Autodesk Inventor part; units mm, degrees
ref_plane "YZ Plane" through (0, 0, 0) normal (1, 0, 0) x (0, 1, 0)
ref_plane "XZ Plane" through (0, 0, 0) normal (0, 1, 0) x (-1, 0, 0)
ref_plane "XY Plane" through (0, 0, 0) normal (0, 0, 1) x (1, 0, 0)
sketch "Szkic1" plane through (0, 0, 0) normal (0, 0, 1) x (1, 0, 0)
  line L0 (-15.1556, -3.6171) -> (-15.1556, -6.6171)
  line L1 (-15.1556, -6.6171) -> (16.3444, -6.6171)
  line L2 (16.3444, -6.6171) -> (16.3444, 13.3829)
  line L3 (16.3444, 13.3829) -> (13.3444, 13.3829)
  line L4 (13.3444, 13.3829) -> (13.3444, -3.6171)
  line L5 (13.3444, -3.6171) -> (-15.1556, -3.6171)
  point P0 (0, 0)
  dimension "d0" = 3
  dimension "d1" = 31.5
  dimension "d2" = 20
  dimension "d3" = 3
extrude "Wyciągnięcie proste1" add sketch "Szkic1" along normal blind 40
fillet "Zaokrąglenie1" radius 3 1 edges at (13.3444, -3.6171, 20)
fillet "Zaokrąglenie3" radius 2 2 edges at (14.8444, 13.3829, 40) (14.8444, 13.3829, 0)
sketch "Szkic4" plane through (-15.1556, -6.6171, 0) normal (0, -1, 0) x (1, 0, 0)
  line L0 (0, 0) -> (31.5, 0)
  line L1 (31.5, 0) -> (31.5, 40)
  line L2 (0, 40) -> (31.5, 40)
  line L3 (0, 0) -> (0, 40)
  line L4 (31.5, 36.2) -> (-0.3213, 36.2)
  line L5 (31.5, 2) -> (31.5, 38)
  line L6 (31.5, 3.8) -> (0, 3.8)
  line L7 (0, 0) -> (0, 40)
  line L8 (27, 36.2) -> (27, 3.8)
  point P0 (15.1556, 0)
  point P1 (23.5, 30)
  point P2 (3.5, 30)
  point P3 (23.5, 10)
  point P4 (3.5, 10)
  dimension "d47" = 32.4
  dimension "d48" = 3.8
  dimension "d50" = 3.5
  dimension "d51" = 3.5
  dimension "d53" = 6.2
  dimension "d54" = 6.2
  dimension "d55" = 6.2
  dimension "d56" = 6.2
  dimension "d68" = 4.5
  dimension "d69" = 3.5
  dimension "d70" = 3.5
  dimension "d78" = 27
sketch "Szkic5" plane through (16.3444, -6.6171, 40) normal (1, 0, 0) x (0, 0, -1)
  arc A0 (40, 18) -> (38, 20) centre (38, 18) ccw
  line L0 (38, 20) -> (2, 20)
  arc A1 (2, 20) -> (0, 18) centre (2, 18) ccw
  line L1 (0, 0) -> (0, 18)
  line L2 (40, 0) -> (0, 0)
  line L3 (40, 0) -> (40, 18)
  point P0 (40, 6.6171)
  point P1 (10, 10)
  point P2 (30, 10)
  dimension "d57" = 10
  dimension "d58" = 10
  dimension "d59" = 10
  dimension "d60" = 10
hole "Otwór3" at (16.3444, 3.3829, 30) at (16.3444, 3.3829, 10) direction (-1, 0, 0) diameter 5 end through all
hole "Otwór4" at (8.3444, -6.6171, 30) at (-11.6556, -6.6171, 30) at (8.3444, -6.6171, 10) at (-11.6556, -6.6171, 10) direction (0, 1, 0) diameter 3 end through all
sketch "Szkic6" plane through (-15.1556, -3.6171, 40) normal (0, 1, 0) x (1, 0, 0)
  circle A0 centre (23.5, 10) radius 1.5
  circle A1 centre (23.5, 30) radius 1.5
  circle A2 centre (23.5, 10) radius 1.5
  circle A3 centre (23.5, 10) radius 3.1
  circle A4 centre (23.5, 30) radius 3.1
  point P0 (15.1556, 40)
  dimension "d79" = 6.2
  dimension "d80" = 6.2
extrude "Wyciągnięcie proste3" cut sketch "Szkic6" along normal blind 10
chamfer "Faza3" distance 4 angle 45 2 edges at (-15.1556, -5.1171, 40) (-15.1556, -5.1171, 0)
fillet "Zaokrąglenie4" radius 2 4 edges at (-15.1556, -5.1171, 36) (-11.1556, -5.1171, 40) (-15.1556, -5.1171, 4) (-11.1556, -5.1171, 0)
properties part number "CNCM_ALU_X_Y_AXis_Mounting_Bracket"
Read the model definition and answer for the solid it produces. Units are mm, in the model's axes. A direction names the side the tool comes from. Give positions to 0.01 mm unless a question says otherwise; leave off trailing zeros. Loops run counter-clockwise (first coordinate to the right, second up) from the corner with the lowest first, then second, coordinate; pieces in that order, holes last. Notation, with made-up numbers: (47, -5) - (99, -5) arc R24 ccw to (99, 33) - close; hole circle Ø1 at (-32, 10.25). An arc over 180 degrees is marked (long way). Answer as CSV lines item,"result". Start each with the question number.
1) Each of these flat-tipped pins is pushed along its axis until it touches: pin 1 Ø2.5 at (x, z) = (8.34, 30) entering from +Y; pin 2 Ø6 at (y, z) = (3.38, 30) entering from +X; pin 3 Ø4 at (y, z) = (7.5, 25) entering from -X; pin 4 Ø5 at (x, z) = (-2, 10) entering from +Y. Where does it stop, or does it pass through?
2) Find section D-D (x = 3.5). Write down the section's boundary in (y, z).
3) Find section C-C (x = -12.5). Write down the section's boundary in (y, z).
4) Straight lines are drawn through the part: L1, parallel to X at y = -5, z = 10; L2, parallel to Y at x = 14.95, z = 10; L3, parallel to X at y = 5.75, z = 38. For each, find the intervals that lie inside material, in ascending order. Write a range as from..to.
5) Determine the mould class of faces 1 (the face through (14.82, 12.81, 0.6)), 2 (the face through (-11.103, -5.138, 0.156)), 3 (the face through (14.8, 3.3, 32.5)) for opening direction Y: released by +Y, released by -Y, zero draft, split by the parting line, or undercut.
6) Find section B-B (z = 19). Write down the section's boundary in (x, y), then the cut area to 3 significant figures.
7) Which of the six approach directions +Z, -Z, +X, -X, +Y, -Y give full straight-line access (tool end or side, diameter ignored) to faces 4 (the face through (15, 13.383, 20)), 5 (the face through (13.344, 6, 20))?
8) Find section A-A (z = 30). Write down the section's boundary in (x, y).
Findings below:
1,pin 1,"through"
1,pin 2,"x = 16.34"
1,pin 3,"x = 13.34"
1,pin 4,"y = -3.62"
2,outline,"(-6.62, 0) - (-3.62, 0) - (-3.62, 40) - (-6.62, 40) - close"
3,outline,"(-6.62, 1.34) - (-3.62, 1.34) - (-3.62, 8.76) - (-6.62, 8.76) - close; (-6.62, 11.24) - (-3.62, 11.24) - (-3.62, 28.76) - (-6.62, 28.76) - close; (-6.62, 31.24) - (-3.62, 31.24) - (-3.62, 38.66) - (-6.62, 38.66) - close"
4,L1,"-15.16..-13.16, -10.16..6.84, 9.84..16.34"
4,L2,"-6.62..0.88, 5.88..13.38"
4,L3,"13.34..16.34"
5,face 1,"released by +Y"
5,face 2,"zero draft"
5,face 3,"undercut"
6,outline,"(-15.16, -6.62) - (16.34, -6.62) - (16.34, 13.38) - (13.34, 13.38) - (13.34, -0.62) arc R3 cw to (10.34, -3.62) - (-15.16, -3.62) - close"
6,area,"147 mm^2"
7,face 4,"+Z, -Z, +X, -X, +Y"
7,face 5,"+Z, -Z, -X, +Y"
8,outline,"(-15.16, -6.62) - (-13.16, -6.62) - (-13.16, -3.62) - (-15.16, -3.62) - close; (-10.16, -6.62) - (6.84, -6.62) - (6.84, -3.62) - (-10.16, -3.62) - close; (9.84, -6.62) - (16.34, -6.62) - (16.34, 0.88) - (13.34, 0.88) - (13.34, -0.62) arc R3 cw to (11.44, -3.41) - (11.44, -3.62) - (9.84, -3.62) - close; (13.34, 5.88) - (16.34, 5.88) - (16.34, 13.38) - (13.34, 13.38) - close"
